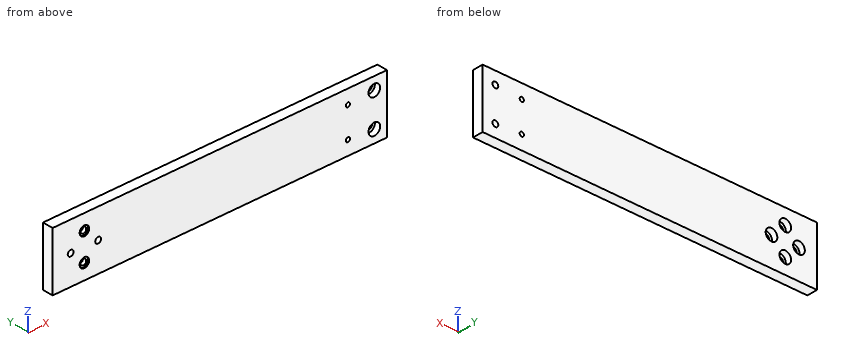
from build123d import *

# Parameters (mm, degrees)
SKETCH1_W           = 316.1
SKETCH1_H           = 55
BOSS_EXTRUDE1_DEPTH = 10
SKETCH2_R           = 2
SKETCH2_R_2         = 2.75
CUT_EXTRUDE1_DEPTH  = 11
SKETCH3_R           = 5.5
CUT_EXTRUDE2_DEPTH  = 5.5
SKETCH4_R           = 2.75
CUT_EXTRUDE3_DEPTH  = 11
SKETCH6_R           = 4.5
CUT_EXTRUDE4_DEPTH  = 1.1
SKETCH7_R           = 5.5
CUT_EXTRUDE5_DEPTH  = 5.5


with BuildPart() as part:
    # Sketch1 → Boss-Extrude1 (new body)
    with BuildSketch(Plane(origin=(0, 0, 0), x_dir=(1, 0, 0), z_dir=(0, 1, 0))):
        with Locations((158.05, 27.5)):
            Rectangle(SKETCH1_W, SKETCH1_H)
    extrude(amount=BOSS_EXTRUDE1_DEPTH)

    # Sketch2 → Cut-Extrude1 (cut, through all)
    with BuildSketch(Plane(origin=(0, 10, 0), x_dir=(1, 0, 0), z_dir=(0, 1, 0))):
        with Locations((279.1, 13.3)):
            Circle(SKETCH2_R)
        with Locations((279.1, 41.7)):
            Circle(SKETCH2_R)
        with Locations((304.1, 43.3)):
            Circle(SKETCH2_R_2)
        with Locations((304.1, 11.7)):
            Circle(SKETCH2_R_2)
    extrude(amount=-CUT_EXTRUDE1_DEPTH, mode=Mode.SUBTRACT)

    # Sketch3 → Cut-Extrude2 (cut)
    with BuildSketch(Plane.XZ):
        with Locations((304.1, -11.7)):
            Circle(SKETCH3_R)
        with Locations((304.1, -43.3)):
            Circle(SKETCH3_R)
    extrude(amount=-CUT_EXTRUDE2_DEPTH, mode=Mode.SUBTRACT)

    # Sketch4 → Cut-Extrude3 (cut, through all)
    with BuildSketch(Plane(origin=(0, 10, 0), x_dir=(1, 0, 0), z_dir=(0, 1, 0))):
        with Locations((17, 27.5)):
            Circle(SKETCH4_R)
        with Locations((30, 40.5)):
            Circle(SKETCH4_R)
        with Locations((43, 27.5)):
            Circle(SKETCH4_R)
        with Locations((30, 14.5)):
            Circle(SKETCH4_R)
    extrude(amount=-CUT_EXTRUDE3_DEPTH, mode=Mode.SUBTRACT)

    # Sketch6 → Cut-Extrude4 (cut)
    with BuildSketch(Plane.XZ):
        with Locations((30, -14.5)):
            Circle(SKETCH6_R)
        with Locations((30, -40.5)):
            Circle(SKETCH6_R)
    extrude(amount=-CUT_EXTRUDE4_DEPTH, mode=Mode.SUBTRACT)

    # Sketch7 → Cut-Extrude5 (cut)
    with BuildSketch(Plane(origin=(0, 10, 0), x_dir=(1, 0, 0), z_dir=(0, 1, 0))):
        with Locations((17, 27.5)):
            Circle(SKETCH7_R)
        with Locations((30, 40.5)):
            Circle(SKETCH7_R)
        with Locations((43, 27.5)):
            Circle(SKETCH7_R)
        with Locations((30, 14.5)):
            Circle(SKETCH7_R)
    extrude(amount=-CUT_EXTRUDE5_DEPTH, mode=Mode.SUBTRACT)


solid = part.part
Read the model definition and answer for the solid it produces. Units are mm, in the model's axes. Round coordinates to 2 decimals unless told otherwise and drop trailing zeros. Write each loop counter-clockwise with the first axis right and the second up, starting at its lowest first coordinate (ties: lowest second). Pieces come first, ordered by that corner, then holes.
1. The part is cut by section A-A, the plane x = 17. Determine the outline of the cut face in (y, z).
2. Straight lines are drawn through the part: L1, parallel to Z at x = 30, y = 5.9; L2, parallel to X at y = 1.45, z = -27.5; L3, parallel to X at y = 6.3, z = -40.5. For each, find the intervals that lie inside material, in ascending order.
3. Given pin 1 Ø6.5 at (x, z) = (304.1, -11.7) entering from -Y; pin 2 Ø4.5 at (x, z) = (279.1, -13.3) entering from -Y; pin 3 Ø10 at (x, z) = (30, -14.5) entering from +Y; pin 4 Ø6.5 at (x, z) = (30, -40.5) entering from -Y, each flat-ended and moving along its own axis, determine where each tip first touches the part or whether it passes through.
4. The part is cut by section B-B, the plane y = 7.25. State how many separate pieces and enclosed holes the cut face has, then the cut area to 3 significant figures.
Values:
1. outline: (0, -55) - (10, -55) - (10, -33) - (4.5, -33) - (4.5, -30.25) - (0, -30.25) - close; (0, -24.75) - (4.5, -24.75) - (4.5, -22) - (10, -22) - (10, 0) - (0, 0) - close
2. L1: z = -55 to -46, -35 to -20, -9 to 0
2. L2: x = 0 to 14.25, 19.75 to 40.25, 45.75 to 316.1
2. L3: x = 0 to 24.5, 35.5 to 277.5, 280.7 to 316.1
3. pin 1: stops at y = 5.5
3. pin 2: stops at y = 0
3. pin 3: stops at y = 4.5
3. pin 4: stops at y = 1.1
4. separate pieces: 1
4. enclosed holes: 8
4. area: 16,900 mm2
